from build123d import *

# Parameters (mm, degrees)
BOSS_EXTRUDE1_DEPTH     = 7.7
SKETCH2_W               = 7
SKETCH2_H               = 3.1
CUT_EXTRUDE1_DEPTH      = 79.027559234
FILLET1_R               = 10
BOSS_EXTRUDE2_DEPTH     = 2
BOSS_EXTRUDE3_DEPTH     = 33.45
BOSS_EXTRUDE4_REACH     = 112.929
CUT_EXTRUDE2_DEPTH      = 111.928772192
CUT_EXTRUDE2_DEPTH_BACK = 111.928772192
CUT_EXTRUDE3_DEPTH      = 10
FILLET3_R               = 1
FILLET4_R               = 5
FILLET5_R               = 3


with BuildPart() as part:
    # Sketch1 → Boss-Extrude1 (new body)
    with BuildSketch(Plane(origin=(0, 0, 0), x_dir=(1, 0, 0), z_dir=(0, 1, 0))):
        Polygon((0, 0), (-16.35, 0), (-16.35, -9.85), (-2.6, -9.85), (-2.6, -33), (-20.1, -33), (-20.1, -75), (0, -75), align=None)
    extrude(amount=BOSS_EXTRUDE1_DEPTH)

    # Sketch2 → Cut-Extrude1 (cut, through all)
    with BuildSketch(Plane.XY.offset(75)):
        with Locations((-16.6, 3.55)):
            Rectangle(SKETCH2_W, SKETCH2_H)
    extrude(amount=-CUT_EXTRUDE1_DEPTH, mode=Mode.SUBTRACT)

    # Fillet1
    fillet1_edges = [part.edges().sort_by_distance(p)[0] for p in [
        (-2.6, 3.85, 33),
    ]]
    fillet(fillet1_edges, radius=FILLET1_R)

    # Sketch3 → Boss-Extrude2 (add)
    with BuildSketch(Plane(origin=(0, 7.7, 0), x_dir=(1, 0, 0), z_dir=(0, 1, 0))):
        Polygon((0, 4.5), (-33.45, 4.5), (-33.45, -75), (-10, -105), (0, -105), align=None)
    extrude(amount=BOSS_EXTRUDE2_DEPTH)

    # Sketch4 → Boss-Extrude3 (add)
    with BuildSketch(Plane(origin=(0, 0, 0), x_dir=(0, 0, -1), z_dir=(1, 0, 0))):
        Polygon((-105, 9.7), (-105, 12.7), (-90, 12.7), (-50.25, 9.7), align=None)
    extrude(amount=-BOSS_EXTRUDE3_DEPTH)

    # Boss-Extrude4: up to this face of the body (flat: up to its plane)
    boss_extrude4_end = Plane(part.part.faces().sort_by_distance((0, 5.848980441, 46.191947566))[0])
    # Sketch5 → Boss-Extrude4 (add, up to the picked face)
    with BuildSketch(Plane.ZY.offset(33.45), mode=Mode.PRIVATE) as boss_extrude4_sk1:
        Polygon((75, 7.7), (75, -5), (82, -5), (105, 7.7), align=None)
    boss_extrude4_tool1 = split(extrude(boss_extrude4_sk1.sketch, amount=-BOSS_EXTRUDE4_REACH, mode=Mode.PRIVATE), bisect_by=boss_extrude4_end, keep=Keep.BOTH, mode=Mode.PRIVATE)
    add(boss_extrude4_tool1.solids().sort_by(Axis((-33.45, 2.665766, 85.441441), (1, 0, 0)))[0])

    # Sketch6 → Cut-Extrude2 (cut, two sides: drawn at the far end of the back side and taken through both)
    with BuildSketch(Plane(origin=(0, 7.7, 0), x_dir=(1, 0, 0), z_dir=(0, 1, 0)).offset(-CUT_EXTRUDE2_DEPTH_BACK)):
        Polygon((-33.45, -75), (-10, -105), (-33.45, -105), align=None)
    extrude(amount=CUT_EXTRUDE2_DEPTH + CUT_EXTRUDE2_DEPTH_BACK, mode=Mode.SUBTRACT)

    # Sketch7 → Cut-Extrude3 (cut)
    with BuildSketch(Plane(origin=(0, 0, 0), x_dir=(0, 0, -1), z_dir=(1, 0, 0))):
        Polygon((-75, 0), (-85, 0), (-80, -5), (-75, -5), align=None)
    extrude(amount=-CUT_EXTRUDE3_DEPTH, mode=Mode.SUBTRACT)

    # Fillet3
    # the kernel refuses this fillet: 1 mm, written as the material it takes off along each edge
    with BuildSketch(Plane(origin=(5.810983209, -5, 80), x_dir=(0, 0, 1), z_dir=(-1, 0, 0))) as fillet3_piece_1:
        with BuildLine():
            CenterArc((2.350701034, 0.936487472), FILLET3_R, 135, 114.469800521)
            Line((1.643594253, 1.643594253), (1.629452117, 1.657736389))
            Line((1.629452117, 1.657736389), (-0.014142136, 0.014142136))
            Line((-0.014142136, 0.014142136), (0, -0.02))
            ThreePointArc((0, -0.02), (1, -0.02), (1.992985979, -0.018729749))
            Line((1.992985979, -0.018729749), (2, 0))
        make_face()
    extrude(amount=15.810983209, mode=Mode.SUBTRACT)
    with BuildSketch(Plane(origin=(-10, -5, 82.5), x_dir=(-1, 0, 0), z_dir=(0, 0, -1))) as fillet3_piece_2_section:
        with BuildLine():
            CenterArc((FILLET3_R, FILLET3_R), FILLET3_R, 180, 90)
            Line((0, FILLET3_R), (-FILLET3_R * 0.02, FILLET3_R))
            Line((-FILLET3_R * 0.02, FILLET3_R), (-FILLET3_R * 0.02, -FILLET3_R * 0.02))
            Line((-FILLET3_R * 0.02, -FILLET3_R * 0.02), (FILLET3_R, -FILLET3_R * 0.02))
            Line((FILLET3_R, -FILLET3_R * 0.02), (FILLET3_R, 0))
        make_face()
    fillet3_piece_2 = extrude(amount=10, mode=Mode.PRIVATE)
    fillet3_piece_2 = split(fillet3_piece_2, bisect_by=Plane(origin=(-10.222841489, -6.700692184, 78.299307816), z_dir=(0, 0.7071067811865466, -0.7071067811865485)), keep=Keep.TOP, mode=Mode.PRIVATE)
    add(fillet3_piece_2, mode=Mode.SUBTRACT)
    with BuildSketch(Plane(origin=(5.810983209, -5, 80), x_dir=(0, 0, 1), z_dir=(-1, 0, 0))) as fillet3_piece_3a_section:
        with BuildLine():
            CenterArc((2.350701034, 0.936487472), FILLET3_R, 135, 114.469800521)
            Line((1.643594253, 1.643594253), (1.629452117, 1.657736389))
            Line((1.629452117, 1.657736389), (-0.014142136, 0.014142136))
            Line((-0.014142136, 0.014142136), (0, -0.02))
            ThreePointArc((0, -0.02), (1, -0.02), (1.992985979, -0.018729749))
            Line((1.992985979, -0.018729749), (2, 0))
        make_face()
    fillet3_piece_3a = extrude(amount=21.621966417, mode=Mode.PRIVATE)
    fillet3_piece_3a = split(fillet3_piece_3a, bisect_by=Plane(origin=(-10, -4.567151235, 80.996776665), z_dir=(-1, 0, 0)), keep=Keep.TOP, mode=Mode.PRIVATE)
    with BuildSketch(Plane(origin=(-10, -5, 82.5), x_dir=(-1, 0, 0), z_dir=(0, 0, -1))) as fillet3_piece_3b_section:
        with BuildLine():
            CenterArc((FILLET3_R, FILLET3_R), FILLET3_R, 180, 90)
            Line((0, FILLET3_R), (-FILLET3_R * 0.02, FILLET3_R))
            Line((-FILLET3_R * 0.02, FILLET3_R), (-FILLET3_R * 0.02, -FILLET3_R * 0.02))
            Line((-FILLET3_R * 0.02, -FILLET3_R * 0.02), (FILLET3_R, -FILLET3_R * 0.02))
            Line((FILLET3_R, -FILLET3_R * 0.02), (FILLET3_R, 0))
        make_face()
    fillet3_piece_3b = extrude(amount=10, mode=Mode.PRIVATE)
    fillet3_piece_3b = split(fillet3_piece_3b, bisect_by=Plane(origin=(-10.238471404, -4.220535034, 80.779464966), z_dir=(0, -0.7071067811865466, 0.7071067811865485)), keep=Keep.TOP, mode=Mode.PRIVATE)
    fillet3_piece_3 = fillet3_piece_3a & fillet3_piece_3b
    add(fillet3_piece_3, mode=Mode.SUBTRACT)

    # Fillet4
    fillet4_edges = [part.edges().sort_by_distance(p)[0] for p in [
        (-33.45, 8.7, -4.5),
    ]]
    fillet(fillet4_edges, radius=FILLET4_R)

    # Mirror1: part across plane


with BuildPart() as part_1:
    add(part.part)
    add(part.part.mirror(Plane(origin=(0, 7.7, 75), x_dir=(0, 0, 1), z_dir=(-1, 0, 0))))

    # Fillet5
    # the kernel refuses this fillet: 3 mm, written as the material it takes off along each edge
    with BuildSketch(Plane(origin=(-38.068859068, -5, 69.091011854), x_dir=(0.7878650861711843, 0, -0.6158478756904764), z_dir=(0.6158478756904763, 0, 0.7878650861711843))) as fillet5_piece_1:
        with BuildLine():
            CenterArc((FILLET5_R, FILLET5_R), FILLET5_R, 180, 90)
            Line((0, FILLET5_R), (0, 0))
            Line((0, 0), (FILLET5_R, 0))
        make_face()
    extrude(amount=23.884769896, mode=Mode.SUBTRACT)
    with BuildSketch(Plane(origin=(38.068859068, -5, 69.091011854), x_dir=(-0.7878650861711843, 0, -0.6158478756904764), z_dir=(-0.6158478756904763, 0, 0.7878650861711843))) as fillet5_piece_2:
        with BuildLine():
            CenterArc((FILLET5_R, -FILLET5_R), FILLET5_R, 90, 90)
            Line((0, -FILLET5_R), (0, 0))
            Line((0, 0), (FILLET5_R, 0))
        make_face()
    extrude(amount=23.884769896, mode=Mode.SUBTRACT)


solid = part_1.part
CAD build for the part. Positions are in the model's coordinates, mm. A direction names the side the tool comes from. Round coordinates to 2 decimals unless told otherwise and drop trailing zeros. Loops run counter-clockwise (first coordinate to the right, second up) from the corner with the lowest first, then second, coordinate; pieces in that order, holes last.
(1) Cut at A-A (z = 6). Give the cut face in (x, y).
(2) Drop flat-ended pins along their axis: pin 1 (8 mm diameter, centred on x = 26, z = 38, fed in from +Y); pin 2 (1 mm diameter, centred on x = 15, z = 7, fed in from -Y); pin 3 (3.5 mm diameter, centred on y = 4, z = 60, fed in from +X). Give the stop position or say it passes through.
(3) Wall check: line 1 along X through (y, z) = (3.25, 52.5); line 2 along Y through (x, z) = (-9, 2.5); line 3 along X through (y, z) = (5.5, 37.5). Give the ranges that are in metal, low to high.
(4) Two-plate mould, pull along Y, no slides. Class faces 1 (the flat face through (20.1, 6, 54)), 2 (the flat face through (10, -2, 79)), 3 (the flat face through (0.36, -0.15, 90.78)): +Y half, -Y half, draft (parallel to the pull), parting line (faces both ways), or undercut.
(5) Cut at C-C (z = 36). Give the cut face in (x, y).
(6) Which spindle directions (+Z, -Z, +X, -X, +Y, -Y) get a long thin tool onto all of the face, cutting with end or side? Do faces 4 (the flat face through (-15, 2, 5)), 5 (the flat face through (-2.6, 4, 16)), 6 (the flat face through (0, 9.7, 22)). Say none if no direction does.
(7) Cut at B-B (y = 3.5). Give the cut face in (x, z).
Findings below:
1. outline: (-33.45, 7.7) - (-16.35, 7.7) - (-16.35, 5.1) - (-13.1, 5.1) - (-13.1, 2) - (-16.35, 2) - (-16.35, 0) - (16.35, 0) - (16.35, 2) - (13.1, 2) - (13.1, 5.1) - (16.35, 5.1) - (16.35, 7.7) - (33.45, 7.7) - (33.45, 9.7) - (-33.45, 9.7) - close
2. pin 1: stops at y = 9.7
2. pin 2: stops at y = 0
2. pin 3: stops at x = 20.1
3. line 1: x = -13.1 to 13.1
3. line 2: y = 0 to 9.7
3. line 3: x = -20.1 to 20.1
4. face 1: draft
4. face 2: undercut
4. face 3: -Y half
5. outline: (-33.45, 7.7) - (-20.1, 7.7) - (-20.1, 5.1) - (-13.1, 5.1) - (-13.1, 2) - (-20.1, 2) - (-20.1, 0) - (20.1, 0) - (20.1, 2) - (13.1, 2) - (13.1, 5.1) - (20.1, 5.1) - (20.1, 7.7) - (33.45, 7.7) - (33.45, 9.7) - (-33.45, 9.7) - close
6. face 4: -Z, -X
6. face 5: -X, -Y
6. face 6: -Z, +X, -X, +Y
7. outline: (-33.45, 75) - (-13.1, 75) - (-13.1, 33) - (-12.6, 33) arc R10 cw to (-2.6, 23) - (-2.6, 9.85) - (-13.1, 9.85) - (-13.1, 0) - (13.1, 0) - (13.1, 9.85) - (2.6, 9.85) - (2.6, 23) arc R10 cw to (12.6, 33) - (13.1, 33) - (13.1, 75) - (33.45, 75) - (15.95, 97.39) - (-15.95, 97.39) - close
